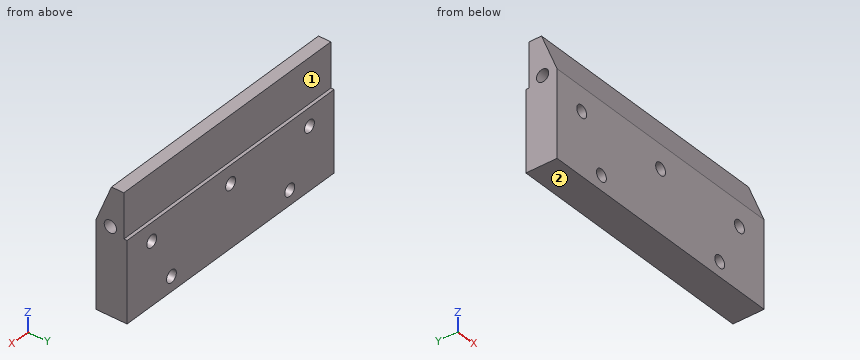
```python
from build123d import *

# Parameters (mm, degrees)
CROQUIS1_W              = 105
CROQUIS1_H              = 50.8
SALIENTE_EXTRUIR1_DEPTH = 12.7
CROQUIS2_W              = 18.097769025
CROQUIS2_H              = 1.305463626
CORTAR_EXTRUIR1_DEPTH   = 109.772468943
CROQUIS3_R              = 2.5
CORTAR_EXTRUIR2_DEPTH   = 60.688357324
CROQUIS4_R              = 2.5
CORTAR_EXTRUIR3_DEPTH   = 60.688357324
CROQUIS5_R              = 2.5
CORTAR_EXTRUIR4_DEPTH   = 12


with BuildPart() as part:
    # Croquis1 → Saliente-Extruir1 (new body)
    with BuildSketch(Plane(origin=(0, 0, 0), x_dir=(1, 0, 0), z_dir=(0, 1, 0))):
        Rectangle(CROQUIS1_W, CROQUIS1_H)
    extrude(amount=SALIENTE_EXTRUIR1_DEPTH)

    # Croquis2 → Cortar-Extruir1 (cut, through all)
    with BuildSketch(Plane(origin=(52.5, 0, 0), x_dir=(0, 0, -1), z_dir=(1, 0, 0))):
        Polygon((-25.4, 6.35), (-9.701031489, 0), (-25.4, 0), align=None)
        with Locations((-16.351115488, 12.047268187)):
            Rectangle(CROQUIS2_W, CROQUIS2_H)
    extrude(amount=-CORTAR_EXTRUIR1_DEPTH, mode=Mode.SUBTRACT)

    # Croquis3 → Cortar-Extruir2 (cut, through all)
    with BuildSketch(Plane(origin=(0, 12.7, 0), x_dir=(1, 0, 0), z_dir=(0, 1, 0))):
        with Locations(Location((0, 0, 0), (0, 0, 270))):
            Circle(CROQUIS3_R)
        with Locations(Location((-40, 0, 0), (0, 0, 270))):
            Circle(CROQUIS3_R)
        with Locations(Location((40, 0, 0), (0, 0, 270))):
            Circle(CROQUIS3_R)
    extrude(amount=-CORTAR_EXTRUIR2_DEPTH, mode=Mode.SUBTRACT)

    # Croquis4 → Cortar-Extruir3 (cut, through all)
    with BuildSketch(Plane(origin=(0, 12.7, 0), x_dir=(1, 0, 0), z_dir=(0, 1, 0))):
        with Locations(Location((-30, 19.4, 0), (0, 0, 270))):
            Circle(CROQUIS4_R)
        with Locations(Location((30, 19.4, 0), (0, 0, 270))):
            Circle(CROQUIS4_R)
    extrude(amount=-CORTAR_EXTRUIR3_DEPTH, mode=Mode.SUBTRACT)

    # Croquis5 → Cortar-Extruir4 (cut)
    with BuildSketch(Plane(origin=(52.5, 0, 0), x_dir=(0, 0, -1), z_dir=(1, 0, 0))):
        with Locations((-9.701031489, 5.890011881)):
            Circle(CROQUIS5_R)
    cortar_extruir4 = extrude(amount=-CORTAR_EXTRUIR4_DEPTH, mode=Mode.SUBTRACT)

    # Simetría1: Cortar-Extruir4 across plane
    add(cortar_extruir4.mirror(Plane(origin=(0, 0, 0), x_dir=(0, 0, 1), z_dir=(1, 0, 0))), mode=Mode.SUBTRACT)


solid = part.part
```
Part model, mm, in its own coordinate system. Face numbers are marked on the shaded views. A direction names the side the tool comes from. Coordinates: 2 decimals unless noted, no trailing zeros. Order: outer loops, then holes, each group sorted by start corner. A loop starts at its lowest first (then second) coordinate and runs counter-clockwise, first axis right, second up. Notation, with made-up numbers: (10.5, -19.5) - (26.5, -19.5) arc R28 ccw to (26.5, 18.5) - close; hole circle Ø10 at (59, 72). An arc over 180 degrees is marked (long way). Return JSON: item names as keys, results as strings. Group by question number.
Item 1: Which spindle directions (+Z, -Z, +X, -X, +Y, -Y) get a long thin tool onto all of the face, cutting with end or side? Do the marked faces 1 and 2. Say none if no direction does.
Item 2: Cut at D-D (x = 31.5). List the corners of the cut face in (y, z).
Item 3: Cut at B-B (z = -19.4). List the corners of the cut face in (x, y).
Item 4: Drill centre lines: probe 1 along X at (y, z) = (3.75, -19.4); probe 2 along X at (y, z) = (6.5, -18); probe 3 along Z at (x, y) = (41, 1). Where is each one in solid material? Low to high. Write a range as from..to.
Item 5: Cut at C-C (z = 0). List the corners of the cut face in (x, y).
Item 6: Pin check, flat tips, straight feed: pin 1 (1 mm diameter, centred on x = 4.5, y = 2, fed in from +Z); pin 2 (4 mm diameter, centred on x = -30, z = -19.4, fed in from +Y); pin 3 (4 mm diameter, centred on x = 7.5, z = 19, fed in from -Y); pin 4 (1 mm diameter, centred on x = 16, y = 12, fed in from +Z). Stop position of each tip, or through.
Item 7: Cut at A-A (x = 0). List the corners of the cut face in (y, z).
Check values:
{
 "1": {"face 1": "+Z, +X, -X, +Y", "face 2": "-Z, +X, -X, +Y, -Y"},
 "2": {"outline": "(0, -25.4) - (12.7, -25.4) - (12.7, -21.4) - (0, -21.4) - close; (0, -17.4) - (12.7, -17.4) - (12.7, 7.3) - (11.39, 7.3) - (11.39, 25.4) - (6.35, 25.4) - (0, 9.7) - close"},
 "3": {"outline": "(-52.5, 0) - (-32.5, 0) - (-32.5, 12.7) - (-52.5, 12.7) - close; (-27.5, 0) - (27.5, 0) - (27.5, 12.7) - (-27.5, 12.7) - close; (32.5, 0) - (52.5, 0) - (52.5, 12.7) - (32.5, 12.7) - close"},
 "4": {"probe 1": "x = -52.5..-32.5, -27.5..27.5, 32.5..52.5", "probe 2": "x = -52.5..-32.07, -27.93..27.93, 32.07..52.5", "probe 3": "z = -25.4..-2.29, 2.29..12.17"},
 "5": {"outline": "(-52.5, 0) - (-42.5, 0) - (-42.5, 12.7) - (-52.5, 12.7) - close; (-37.5, 0) - (-2.5, 0) - (-2.5, 12.7) - (-37.5, 12.7) - close; (2.5, 0) - (37.5, 0) - (37.5, 12.7) - (2.5, 12.7) - close; (42.5, 0) - (52.5, 0) - (52.5, 12.7) - (42.5, 12.7) - close"},
 "6": {"pin 1": "stops at z = 15.88", "pin 2": "passes through", "pin 3": "stops at y = 2.95", "pin 4": "stops at z = 7.3"},
 "7": {"outline": "(0, -25.4) - (12.7, -25.4) - (12.7, -2.5) - (0, -2.5) - close; (0, 2.5) - (12.7, 2.5) - (12.7, 7.3) - (11.39, 7.3) - (11.39, 25.4) - (6.35, 25.4) - (0, 9.7) - close"}
}
